```python
from build123d import *

# Parameters (mm, degrees)
F0_R     = 6
F1_DEPTH = 4.7
F2_R     = 1.6
F3_DEPTH = 25


with BuildPart() as f1:
    # F0 (on Top) → F1 (new body)
    with BuildSketch(Plane.XY):
        Circle(F0_R)
    extrude(amount=F1_DEPTH)

    # F2 (on face) → F3 (cut)
    with BuildSketch(Plane.XY.offset(4.7)):
        Circle(F2_R)
    extrude(amount=-F3_DEPTH, mode=Mode.SUBTRACT)

    # F4 (on Front) → F5 (revolve, cut)
    with BuildSketch(Plane.XZ):
        with BuildLine():
            Line((0, 2.5), (0, 12.5))
            ThreePointArc((0, 12.5), (-5, 7.5), (0, 2.5))
        make_face()
    revolve(axis=Axis((0, 0, 7.5), (0, 0, -1)), mode=Mode.SUBTRACT)


solid = f1.part
```
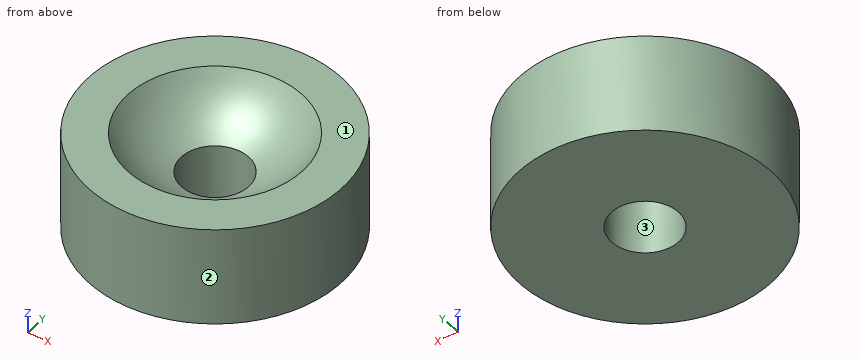
Source: CAD feature listing. Evaluate the final solid. Frame: model axes, mm. Face numbers are marked on the shaded views. Coordinates: 2 decimals unless noted, no trailing zeros. Loops run counter-clockwise (first coordinate to the right, second up) from the corner with the lowest first, then second, coordinate; pieces in that order, holes last. Notation, with made-up numbers: M -39.75,-30.75 L 18.25,-30.75 A20 ccw 18.25,-4.75 Z; hole C 83,54 d6. An arc over 180 degrees is marked long. Put each result on its own line as item: value. Start each with the question number.
1) Cut plane D-D on y = -3. Return the cut outline in (x, z), then the cut area to 3 significant figures.
2) Pull-direction query (Y, two-part tool) for the marked faces 1, 2 and 3; classes: pulls with the +Y half, pulls with the -Y half, needs draft (parallel to the pull), parting line crosses it, or undercut.
3) Contact query for flat-ended pins moving along their axis: pin 1 Ø5 at (x, y) = (1, 2.5) entering from -Z; pin 2 Ø1 at (y, z) = (3.5, 1) entering from +X; pin 3 Ø3.5 at (x, y) = (0, 0) entering from +Z. Output: stop coordinate, or through.
4) Cut plane A-A on x = 0. Return the cut outline in (y, z).
5) Cut plane C-C on z = 2.55. Return the cut outline in (x, y), then the cut area to 3 significant figures.
6) Ray query, L1, parallel to Y at x = 0, z = 2.05; L2, parallel to Y at x = 0.5, z = 1.2; L3, parallel to X at y = 2.25, z = 4.2. Return the intervals inside material, ascending. Write a range as from..to.
The answers:
1. outline: M -5.2,0 L 5.2,0 L 5.2,4.7 L 2.86,4.7 A4 cw -2.86,4.7 L -5.2,4.7 Z
1. area: 44.1 mm²
2. face 1: needs draft
2. face 2: parting line crosses it
2. face 3: undercut
3. pin 1: stops at z = 0
3. pin 2: stops at x = 5.2
3. pin 3: stops at z = 2.82
4. outline: M -6,0 L -1.6,0 L -1.6,2.76 A5 cw -4.14,4.7 L -6,4.7 Z; M 1.6,0 L 6,0 L 6,4.7 L 4.14,4.7 A5 cw 1.6,2.76 Z
5. outline: C 0,0 d12; hole C 0,0 d3.2
5. area: 105 mm²
6. L1: y = -6..-1.6, 1.6..6
6. L2: y = -5.98..-1.52, 1.52..5.98
6. L3: x = -5.56..-3.01, 3.01..5.56
